Input: dimensioned drawing with shaded views. Units: mm. Origin: part minimum x, y, z. A direction names the side the tool comes from. Give positions to 0.01 mm unless a question says otherwise; leave off trailing zeros. Order: outer loops, then holes, each group sorted by start corner. A loop starts at its lowest first (then second) coordinate and runs counter-clockwise, first axis right, second up.
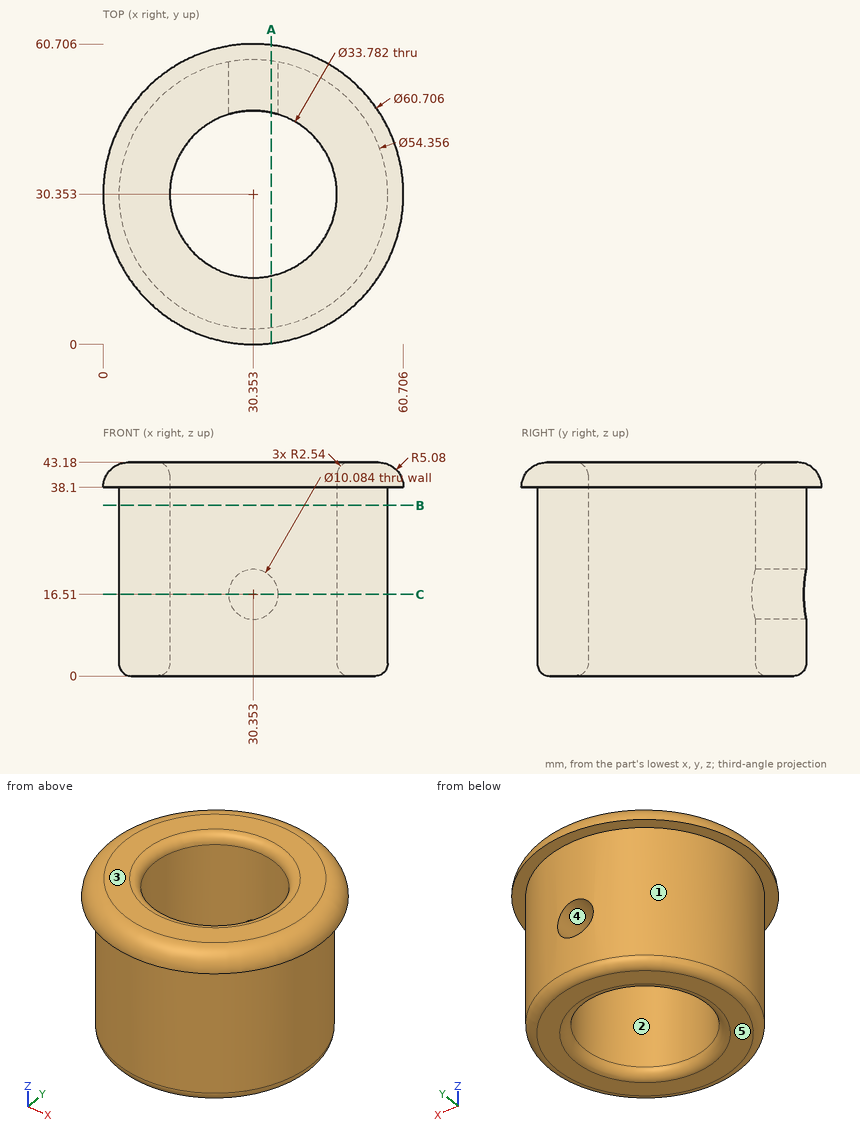
1) Material intervals for L1, parallel to X at y = 51.5, z = 16.51 (1 decimal); L2, parallel to Y at x = 25.5, z = 19; L3, parallel to Y at x = 31.5, z = 40 (1 decimal), sorted ascending.
Report:
L1: x = 13.3 to 25.3, 35.4 to 47.4
L2: y = 3.61 to 14.17, 46.53 to 57.09
L3: y = 0.4 to 13.5, 47.2 to 60.3
2) Section query C-C, the plane z = 16.51. Return the cut outline in (x, y) (1 decimal).
Report:
outline: (25.3, 46.5) - (25.3, 57.1) arc R27.2 ccw (long way) to (35.4, 57.1) - (35.4, 46.5) arc R16.9 cw (long way) to start
3) Reachability of the marked faces 4 and 5 from +Z, -Z, +X, -X, +Y, -Y: full face, straight path, thin tool, end or side. Return the list, or none.
Report:
face 4: +Y
face 5: -Z, +X, -X, +Y, -Y
4) Section query A-A, the plane x = 34. Count the separate pieces of the cut face and the enclosed holes in it, and give its area (3 significant figures).
Report:
separate pieces: 3
enclosed holes: 0
area: 842 mm2
5) Section query B-B, the plane z = 34.5. Return the cut outline in (x, y), and give its area (3 significant figures).
Report:
outline: circle Ø54.36 at (30.35, 30.35); hole circle Ø33.78 at (30.35, 30.35)
area: 1,420 mm2
6) Pin query (flat end, axial travel): pin 1 (1 mm diameter, centred on x = 37, z = 9, fed in from -Y); pin 2 (11.5 mm diameter, centred on x = 30.353, z = 16.51, fed in from -Y) (3 decimals); pin 3 (2 mm diameter, centred on y = 24.5, z = 23.5, fed in from +X). Return the tip coordinate at first contact, or that it passes through.
Report:
pin 1: stops at y = 3.88
pin 2: stops at y = 3.175
pin 3: stops at x = 57.09
7) Draft query along X for the marked faces 1, 2 and 3. Return one class per face: +X half, -X half, draft (parallel to the pull), parting line (faces both ways), or undercut.
Report:
face 1: parting line
face 2: undercut
face 3: draft
